The drawing under review shows one solid part. Ordinate dimensions are in mm from its lowest x, y, z. Coordinates: 2 decimals unless noted, no trailing zeros. Loops run counter-clockwise (first coordinate to the right, second up) from the corner with the lowest first, then second, coordinate; pieces in that order, holes last. Notation, with made-up numbers: M 73.5,7.5 L 131.5,7.5 A24 cw 131.5,32.5 Z; hole C 37,-5.75 d8. An arc over 180 degrees is marked long. Answer as a JSON object with one key per item and string values. Group by question number.
1. Consider section C-C (x = 1.75). State the section outline as (y, z) points, then the cut area to 3 significant figures.
2. Consider section A-A (x = 7.75). State the section outline as (y, z) points.
3. To check wall thickness, follow probe 1 along Y at (x, z) = (5.5, 1.75) (1 decimal); probe 2 along Y at (x, z) = (3.5, 2.25) (1 decimal); probe 3 along Y at (x, z) = (3.25, 2.25). State the ranges of each line that lie inside material, in increasing order.
4. Insertion check: pin 1 (1 mm diameter, centred on x = 2, z = 3.5, fed in from +Y). The pin has a flat end and moves straight along its axis. Give the tip position at first contact, or say it passes through.
5. Draft analysis for pull direction Y (two halves, no side actions). For the marked faces 1, 2, 3 and 4, state which applies: +Y half, -Y half, draft (parallel to the pull), parting line (faces both ways), or undercut.
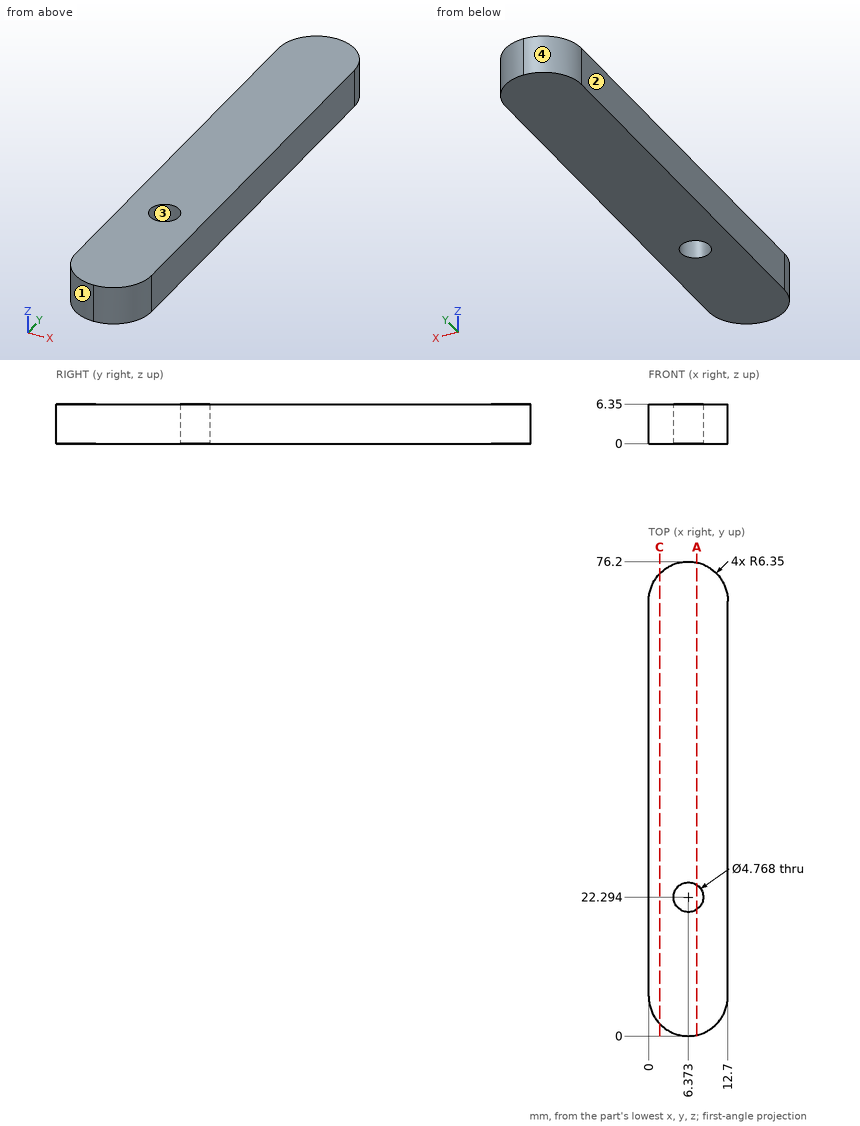
Findings below:
{
 "1": {"outline": "M 1.97,0 L 74.23,0 L 74.23,6.35 L 1.97,6.35 Z", "area": "459 mm^2"},
 "2": {"outline": "M 0.16,0 L 20.35,0 L 20.35,6.35 L 0.16,6.35 Z; M 24.24,0 L 76.04,0 L 76.04,6.35 L 24.24,6.35 Z"},
 "3": {"probe 1": "y = 0.1 to 20.1, 24.5 to 76.1", "probe 2": "y = 0.7 to 75.5", "probe 3": "y = 0.81 to 75.39"},
 "4": {"pin 1": "stops at y = 74.9"},
 "5": {"face 1": "-Y half", "face 2": "draft", "face 3": "undercut", "face 4": "+Y half"}
}
